from build123d import *

# Parameters (mm, degrees)
PAD_DEPTH       = 3
SKETCH002_R     = 2
SKETCH002_R_2   = 1
POCKET_DEPTH    = 3
POCKET001_DEPTH = 3
SKETCH005_R     = 2.33
PAD001_DEPTH    = 10
PAD002_DEPTH    = 3
SKETCH009_R     = 10
SKETCH009_R_2   = 8
PAD003_DEPTH    = 3
SKETCH011_R     = 0.75
POCKET002_DEPTH = 3
PAD004_DEPTH    = 3
SKETCH007_R     = 1.5
POCKET003_DEPTH = 7
POCKET004_DEPTH = 6
SKETCH014_W     = 3.5
SKETCH014_H     = 2
POCKET005_DEPTH = 3
POCKET006_DEPTH = 3
SKETCH013_W     = 6
SKETCH013_H     = 2
POCKET007_DEPTH = 3
SKETCH012_W     = 4.5
SKETCH012_H     = 2
POCKET008_DEPTH = 3


with BuildPart() as part:
    # Sketch001 → Pad (new body)
    with BuildSketch(Plane.XY):
        with BuildLine():
            Line((28.284271, 42.426407), (5.303301, 22.98097))
            Line((5.303301, 22.98097), (0, 22.98097))
            Line((0, 22.98097), (0, 0))
            Line((0, 0), (22.98097, 0))
            Line((22.98097, 0), (22.98097, 5.303301))
            Line((22.98097, 5.303301), (42.426407, 28.284271))
            ThreePointArc((42.426407, 28.284271), (42.426407, 42.426407), (28.284271, 42.426407))
        make_face()
    extrude(amount=PAD_DEPTH)

    # Sketch002 → Pocket (cut)
    with BuildSketch(Plane.XY.offset(3)):
        with Locations((35.355339, 35.355339)):
            Circle(SKETCH002_R)
        with Locations((38.53732, 38.53732)):
            Circle(SKETCH002_R_2)
        with Locations((32.173359, 38.53732)):
            Circle(SKETCH002_R_2)
        with Locations((32.173359, 32.173359)):
            Circle(SKETCH002_R_2)
        with Locations((38.53732, 32.173359)):
            Circle(SKETCH002_R_2)
    extrude(amount=-POCKET_DEPTH, mode=Mode.SUBTRACT)

    # Sketch003 → Pocket001 (cut)
    with BuildSketch(Plane.XY.offset(3)):
        Polygon((20.152543, 8.131728), (8.131728, 20.152543), (11.185273, 22.736312), (22.736312, 11.185273), align=None)
        Polygon((24.028197, 12.712046), (12.712046, 24.028197), (16.528977, 27.257908), (27.257908, 16.528977), align=None)
        Polygon((28.549792, 18.05575), (18.05575, 28.549792), (23.452375, 33.116168), (33.116168, 23.452375), align=None)
    extrude(amount=-POCKET001_DEPTH, mode=Mode.SUBTRACT)

    # Sketch005 → Pad001 (new body)
    with BuildSketch(Plane.XY.offset(3)):
        with Locations((10, 10)):
            Circle(SKETCH005_R)
    extrude(amount=PAD001_DEPTH)

    # Sketch004 → Pad002 (new body)
    with BuildSketch(Plane.XY.offset(3)):
        with BuildLine():
            Line((5.303301, 22.98097), (20.152543, 8.131728))
            ThreePointArc((17.324116, 8.131728), (18.73833, 7.545942), (20.152543, 8.131728))
            Line((17.324116, 8.131728), (4.474874, 20.98097))
            Line((0, 20.98097), (4.474874, 20.98097))
            Line((0, 22.98097), (0, 20.98097))
            Line((5.303301, 22.98097), (0, 22.98097))
        make_face()
        with BuildLine():
            Line((22.98097, 5.303301), (22.98097, 0))
            Line((22.98097, 0), (20.98097, 0))
            Line((20.98097, 0), (17.98097, 0))
            Line((17.98097, 0), (15.98097, 0))
            ThreePointArc((19.48097, 3.5), (17.006097, 2.474874), (15.98097, 0))
            ThreePointArc((19.48097, 3.5), (21.449594, 3.977326), (22.98097, 5.303301))
        make_face()
    extrude(amount=PAD002_DEPTH)

    # Sketch009 → Pad003 (new body)
    with BuildSketch(Plane.XY.offset(3)):
        with Locations((35.355339, 35.355339)):
            Circle(SKETCH009_R)
        with Locations((35.355339, 35.355339)):
            Circle(SKETCH009_R_2, mode=Mode.SUBTRACT)
    extrude(amount=PAD003_DEPTH)

    # Sketch011 → Pocket002 (cut)
    with BuildSketch(Plane.XY.offset(3)):
        with Locations((35.732096, 23.469065)):
            Circle(SKETCH011_R)
    extrude(amount=-POCKET002_DEPTH, mode=Mode.SUBTRACT)

    # Sketch006 → Pad004 (new body)
    with BuildSketch(Plane.XY.offset(3)):
        Polygon((35.944595, 20.623948), (33.360826, 17.570403), (30.532399, 20.39883), (33.116168, 23.452375), align=None)
        Polygon((24.041631, 12.727922), (26.870058, 9.899495), (29.453827, 12.95304), (26.6254, 15.781467), align=None)
    extrude(amount=PAD004_DEPTH)

    # Sketch007 → Pocket003 (cut)
    with BuildSketch(Plane.XY.offset(13)):
        with Locations((10, 10)):
            Circle(SKETCH007_R)
    extrude(amount=-POCKET003_DEPTH, mode=Mode.SUBTRACT)

    # Sketch008 → Pocket004 (cut)
    with BuildSketch(Plane.XY.offset(6)):
        with BuildLine():
            ThreePointArc((21.08097, 0), (19.48097, 1.6), (17.88097, 0))
            Line((21.08097, 0), (17.88097, 0))
        make_face()
    extrude(amount=-POCKET004_DEPTH, mode=Mode.SUBTRACT)

    # Sketch014 → Pocket005 (cut)
    with BuildSketch(Plane.XY.offset(6)):
        with Locations((1.75, 21.98097)):
            Rectangle(SKETCH014_W, SKETCH014_H)
    extrude(amount=-POCKET005_DEPTH, mode=Mode.SUBTRACT)

    # Sketch010 → Pocket006 (cut)
    with BuildSketch(Plane.XY.offset(6)):
        with BuildLine():
            ThreePointArc((33.355339, 27.609372), (35.355339, 27.355339), (37.355339, 27.609372))
            Line((37.355339, 27.609372), (37.355339, 25.55738))
            ThreePointArc((33.355339, 25.55738), (35.355339, 25.355339), (37.355339, 25.55738))
            Line((33.355339, 27.609372), (33.355339, 25.55738))
        make_face()
    extrude(amount=-POCKET006_DEPTH, mode=Mode.SUBTRACT)

    # Sketch013 → Pocket007 (cut)
    with BuildSketch(Plane(origin=(10.777283, -9.119239, 0), x_dir=(0.645942, 0.763386, 0), z_dir=(0.763386, -0.645942, 0))):
        with Locations((27, 4)):
            Rectangle(SKETCH013_W, SKETCH013_H)
    extrude(amount=-POCKET007_DEPTH, mode=Mode.SUBTRACT)

    # Sketch012 → Pocket008 (cut)
    with BuildSketch(Plane(origin=(7.734285, -6.544395, 0), x_dir=(-0.645942, -0.763386, 0), z_dir=(-0.763386, 0.645942, 0))):
        with Locations((-37.25, 4)):
            Rectangle(SKETCH012_W, SKETCH012_H)
    extrude(amount=-POCKET008_DEPTH, mode=Mode.SUBTRACT)


solid = part.part
Could you check a few things on this model? Use its own coordinates, in mm. A direction names the side the tool comes from. Round coordinates to 2 decimals unless told otherwise and drop trailing zeros. Write each loop counter-clockwise with the first axis right and the second up, starting at its lowest first coordinate (ties: lowest second). Pieces come first, ordered by that corner, then holes. Notation, with made-up numbers: (34, -4) - (42, -4) arc R15 cw to (42, 15) - close; hole circle Ø8 at (77, 26). An arc over 180 degrees is marked (long way). Use a Markdown table: item, result.
Q1. I want a section at A-A (x = 10). List the corners of the cut face in (y, z) for me.
Output values:
| item | result |
|---|---|
| outline | (0, 0) - (18.28, 0) - (18.28, 6) - (15.46, 6) - (15.46, 3) - (12.33, 3) - (12.33, 13) - (11.5, 13) - (11.5, 6) - (8.5, 6) - (8.5, 13) - (7.67, 13) - (7.67, 3) - (0, 3) - close; (21.73, 0) - (26.96, 0) - (26.96, 3) - (21.73, 3) - close |
Q2. I want a section at B-B (z = 1.5). Count the separate pieces of the cut face and the enclosed holes in it, plus the area to 3 significant figures.
Output values:
| item | result |
|---|---|
| separate pieces | 1 |
| enclosed holes | 9 |
| area | 929 mm2 |
Q3. For faces 1 (the flat face through (12, 15, 6)), 2 (the flat face through (25.352, 14.276, 4.479)), 3 (the flat face through (22.981, 3, 3)), which set-ups out of +Z, -Z, +X, -X, +Y, -Y let a thin tool reach every point of the face, with its end or its side?
Output values:
| item | result |
|---|---|
| face 1 | +Z, +X, +Y |
| face 2 | +Z, -Z |
| face 3 | +Z, -Z, +X, -Y |
Q4. For pin 1 (5 mm diameter, centred on x = 24.5, y = 28, fed in from +Z); pin 2 (4.5 mm diameter, centred on x = 16, y = 14.5, fed in from +Z); pin 3 (2.5 mm diameter, centred on y = 26, z = 5, fed in from +X); pin 4 (0.8 mm diameter, centred on x = 4, z = 4, fed in from -Y), each with a flat end and sliding along its axis, tell me the tip position at first contact or that it passes through.
Output values:
| item | result |
|---|---|
| pin 1 | through |
| pin 2 | z = 6 |
| pin 3 | x = 41.21 |
| pin 4 | y = 20.98 |
Q5. Please list where these lines run through material, in increasing order: L1, parallel to X at y = 20, z = 2.5; L2, parallel to X at y = 22, z = 2; L3, parallel to Y at x = 39, z = 5.25.
Output values:
| item | result |
|---|---|
| L1 | 0 to 8.28, 13.92 to 16.74, 23.79 to 26.61, 30.19 to 35.42 |
| L2 | 0 to 10.32, 11.92 to 14.74, 21.79 to 24.61, 31.89 to 37.11 |
| L3 | 26.04 to 28.23, 42.48 to 44.67 |
Q6. I want a section at C-C (z = 10). List the corners of the cut face in (x, y) for me, plus the area to 3 significant figures.
Output values:
| item | result |
|---|---|
| outline | circle Ø4.66 at (10, 10); hole circle Ø3 at (10, 10) |
| area | 9.99 mm2 |
Q7. Thinking about a two-plate mould opening in Y: for faces 4 (the cylindrical face through (19.5, 1.6, 3)), 5 (the flat face through (18.45, 18.29, 1.52)), 6 (the flat face through (20, 2, 6)), which applies, released by +Y, released by -Y, zero draft, split by the parting line, or undercut?
Output values:
| item | result |
|---|---|
| face 4 | released by -Y |
| face 5 | undercut |
| face 6 | zero draft |
